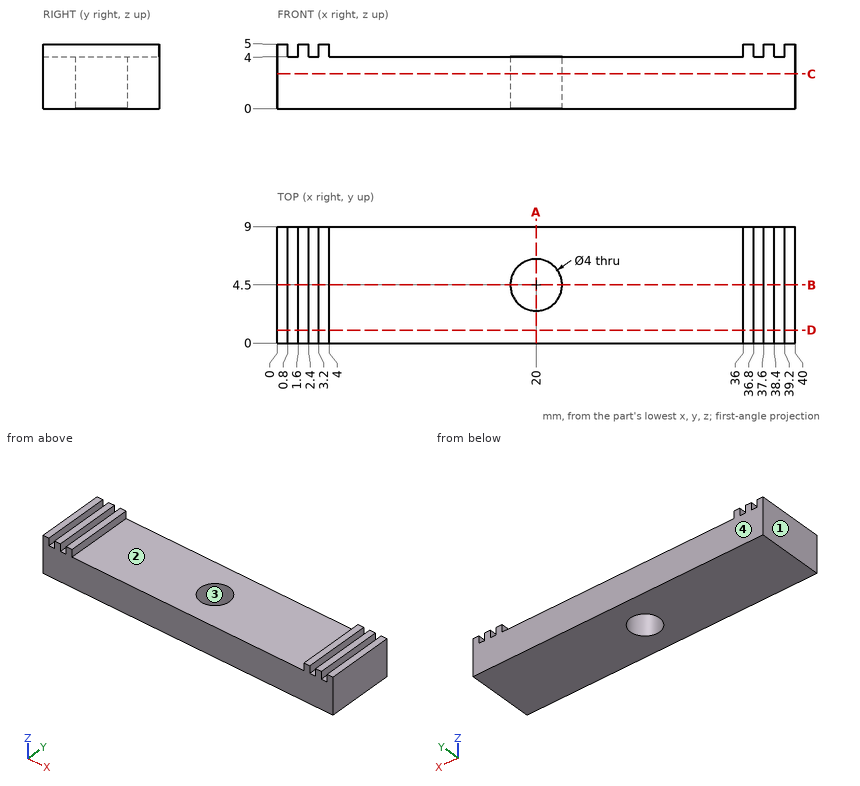
Source: three-view drawing plus pictorial views. Frame: mm from the lowest corner of the part. Give positions to 0.01 mm unless a question says otherwise; leave off trailing zeros. Write each loop counter-clockwise with the first axis right and the second up, starting at its lowest first coordinate (ties: lowest second). Pieces come first, ordered by that corner, then holes. Notation, with made-up numbers: (73.25, 4.25) - (123.25, 4.25) arc R18 cw to (123.25, 31.25) - close; hole circle Ø7 at (50.5, 87). An arc over 180 degrees is marked (long way). Write item = value, one per line. Start each with the question number.
Q1. Draft query along X for the marked faces 1, 2, 3 and 4. Return one class per face: +X half, -X half, draft (parallel to the pull), parting line (faces both ways), or undercut.
Q2. Cut plane D-D, the plane y = 1. Return loops of the section in (x, z), then the cut area to 3 significant figures.
Q3. Cut plane B-B, the plane y = 4.5. Return loops of the section in (x, z).
Q4. Material intervals for probe 1 along X at (y, z) = (6, 4.55); probe 2 along Y at (x, z) = (20, 1.9); probe 3 along Z at (x, y) = (7.5, 2), sorted ascending.
Q5. Pin query (flat end, axial travel): pin 1 Ø2.5 at (x, y) = (16, 3) entering from +Z; pin 2 Ø2.5 at (x, y) = (20, 4.5) entering from -Z. Return the tip coordinate at first contact, or that it passes through.
Q6. Cut plane A-A, the plane x = 20. Return loops of the section in (y, z).
Q7. Cut plane C-C, the plane z = 2.7. Return loops of the section in (x, y), then the cut area to 3 significant figures.
Computed values:
q1.face_1 = -X half
q1.face_2 = undercut
q1.face_3 = undercut
q1.face_4 = draft
q2.outline = (0, 0) - (40, 0) - (40, 5) - (39.2, 5) - (39.2, 4) - (38.4, 4) - (38.4, 5) - (37.6, 5) - (37.6, 4) - (36.8, 4) - (36.8, 5) - (36, 5) - (36, 4) - (4, 4) - (4, 5) - (3.2, 5) - (3.2, 4) - (2.4, 4) - (2.4, 5) - (1.6, 5) - (1.6, 4) - (0.8, 4) - (0.8, 5) - (0, 5) - close
q2.area = 165 mm²
q3.outline = (0, 0) - (18, 0) - (18, 4) - (4, 4) - (4, 5) - (3.2, 5) - (3.2, 4) - (2.4, 4) - (2.4, 5) - (1.6, 5) - (1.6, 4) - (0.8, 4) - (0.8, 5) - (0, 5) - close; (22, 0) - (40, 0) - (40, 5) - (39.2, 5) - (39.2, 4) - (38.4, 4) - (38.4, 5) - (37.6, 5) - (37.6, 4) - (36.8, 4) - (36.8, 5) - (36, 5) - (36, 4) - (22, 4) - close
q4.probe_1 = 0 to 0.8, 1.6 to 2.4, 3.2 to 4, 36 to 36.8, 37.6 to 38.4, 39.2 to 40
q4.probe_2 = 0 to 2.5, 6.5 to 9
q4.probe_3 = 0 to 4
q5.pin_1 = 4
q5.pin_2 = through
q6.outline = (0, 0) - (2.5, 0) - (2.5, 4) - (0, 4) - close; (6.5, 0) - (9, 0) - (9, 4) - (6.5, 4) - close
q7.outline = (0, 0) - (40, 0) - (40, 9) - (0, 9) - close; hole circle Ø4 at (20, 4.5)
q7.area = 347 mm²
